from build123d import *

# Parameters (mm, degrees)
F0_W     = 63.8628005981
F0_H     = 109.5097213984
F1_DEPTH = 20
F2_W     = 47.8628005981
F2_H     = 93.5097213984
F3_DEPTH = 10
F4_W     = 54.004792124
F4_H     = 99.651709199
F4_W_2   = 47.8628005981
F4_H_2   = 93.5097213984
F5_DEPTH = 3


with BuildPart() as f1:
    # F0 (on Top) → F1 (new body)
    with BuildSketch(Plane.XY):
        Rectangle(F0_W, F0_H)
    extrude(amount=F1_DEPTH)

    # F2 (on face) → F3 (cut)
    with BuildSketch(Plane.XY.offset(20)):
        Rectangle(F2_W, F2_H)
    extrude(amount=-F3_DEPTH, mode=Mode.SUBTRACT)

    # F4 (on face) → F5 (join)
    with BuildSketch(Plane.XY.offset(20)):
        Rectangle(F4_W, F4_H)
        Rectangle(F4_W_2, F4_H_2, mode=Mode.SUBTRACT)
    extrude(amount=F5_DEPTH)


solid = f1.part
Verification items for the finished model (mm, model axes). A direction names the side the tool comes from. Round coordinates to 2 decimals unless told otherwise and drop trailing zeros. Order: outer loops, then holes, each group sorted by start corner. A loop starts at its lowest first (then second) coordinate and runs counter-clockwise, first axis right, second up.
1. Access from +Z, -Z, +X, -X, +Y, -Y to the whole of each face (thin tool, end or side, straight path). Record for faces 1 (the flat face through (-23.931, -1, 16)), 2 (the flat face through (27.002, -1, 21)), 3 (the flat face through (-27.002, -1, 21)), 4 (the flat face through (0, 49.826, 21)).
Final values:
face 1: +Z
face 2: +Z, +X, +Y, -Y
face 3: +Z, -X, +Y, -Y
face 4: +Z, +X, -X, +Y
2. Section check A-A on z = 11.5. Record the cut outline in (x, y), then the cut area to 3 significant figures.
Final values:
outline: (-31.93, -54.75) - (31.93, -54.75) - (31.93, 54.75) - (-31.93, 54.75) - close; hole (-23.93, -46.75) - (23.93, -46.75) - (23.93, 46.75) - (-23.93, 46.75) - close
area: 2,520 mm2
3. Thickness scan on L1, parallel to Y at x = 6.5, z = 17; L2, parallel to X at y = -4, z = 16; L3, parallel to X at y = -9, z = 21.25. Record the ranges inside material, lowest first.
Final values:
L1: y = -54.75 to -46.75, 46.75 to 54.75
L2: x = -31.93 to -23.93, 23.93 to 31.93
L3: x = -27 to -23.93, 23.93 to 27
4. Go/stop test with flat-tipped pins: P1, Ø1.5, axis at y = 21, z = 21.5, coming from the -X side; P2, Ø2.5, axis at x = -10.5, z = 22, coming from the -Y side; P3, Ø14.5, axis at x = 6, y = 15, coming from the +Z side. Record where each tip stops, or that it passes through.
Final values:
P1: stops at x = -27
P2: stops at y = -49.83
P3: stops at z = 10
5. Section check B-B on x = -15. Record the cut outline in (y, z).
Final values:
outline: (-54.75, 0) - (54.75, 0) - (54.75, 20) - (49.83, 20) - (49.83, 23) - (46.75, 23) - (46.75, 10) - (-46.75, 10) - (-46.75, 23) - (-49.83, 23) - (-49.83, 20) - (-54.75, 20) - close
6. Section check C-C on y = -27.5. Record the cut outline in (x, z).
Final values:
outline: (-31.93, 0) - (31.93, 0) - (31.93, 20) - (27, 20) - (27, 23) - (23.93, 23) - (23.93, 10) - (-23.93, 10) - (-23.93, 23) - (-27, 23) - (-27, 20) - (-31.93, 20) - close
7. Release check for a two-part mould opening along X. For faces 5 (the flat face through (-31.931, -1, 10)), 6 (the flat face through (0, 46.755, 16)), 7 (the flat face through (0, -54.755, 10)) record: +X half, -X half, draft (parallel to the pull), parting line (faces both ways), or undercut.
Final values:
face 5: -X half
face 6: undercut
face 7: draft
